```python
from build123d import *

# Parameters (mm, degrees)
F0_W         = 95.0192604214
F0_H         = 18.9093053341
F1_DEPTH     = 1.6002
F2_R         = 1.27
F3_DEPTH     = 25.4
F4_R         = 1.27
F5_DEPTH     = 2.54
F6_W         = 48.927821219
F6_H         = 30.7276230305
F7_DEPTH     = 3.6195
F8_T1_DEPTH  = 30.6197
F8_T6_DEPTH  = 56.1276230305
F8_T12_DEPTH = 56.1276230305
F8_T18_DEPTH = 56.1276230305
F8_T25_DEPTH = 56.1276230305
F8_T31_DEPTH = 56.1276230305
F8_T37_DEPTH = 56.1276230305
F8_T43_DEPTH = 56.1276230305
F8_T49_DEPTH = 56.1276230305
F8_T56_DEPTH = 56.1276230305
F8_T62_DEPTH = 56.1276230305
F9_T1_DEPTH  = 37.4142992276
F10_R        = 12.7


# Not quite as in the source:
# - a fillet or chamfer that OpenCascade refuses, or shapes differently, is made with other operations: its cross-section is extruded or revolved along the edge and cut away or added


with BuildPart() as f1:
    # F0 (on Top) → F1 (new body)
    with BuildSketch(Plane.XY):
        Polygon((-24.4639106095, -15.3638115153), (24.4639106095, -15.3638115153), (24.4639106095, -9.454652667), (24.4639106095, 9.454652667), (24.4639106095, 15.3638115153), (-24.4639106095, 15.3638115153), (-24.4639106095, 9.454652667), (-24.4639106095, -9.454652667), align=None)
        with Locations((71.9735408202, 0)):
            Rectangle(F0_W, F0_H)
        with Locations((-71.9735408202, 0)):
            Rectangle(F0_W, F0_H)
    extrude(amount=F1_DEPTH)

    # F2 (on face) → F3 (cut)
    with BuildSketch(Plane.XY.offset(1.6002)):
        with Locations((106.7831710309, 0)):
            Circle(F2_R)
        with Locations((94.0831710309, 0)):
            Circle(F2_R)
        with Locations((81.3831710309, 0)):
            Circle(F2_R)
        with Locations((68.6831710309, 0)):
            Circle(F2_R)
        with Locations((55.9831710309, 0)):
            Circle(F2_R)
        with Locations((43.2831710309, 0)):
            Circle(F2_R)
    extrude(amount=-F3_DEPTH, mode=Mode.SUBTRACT)

    # F4 (on face) → F5 (join)
    with BuildSketch(Plane.XY.offset(1.6002)):
        with Locations((-106.7719441229, 0)):
            Circle(F4_R)
        with Locations((-94.0719441229, 0)):
            Circle(F4_R)
        with Locations((-81.3719441229, 0)):
            Circle(F4_R)
        with Locations((-68.6719441229, 0)):
            Circle(F4_R)
        with Locations((-55.9719441229, 0)):
            Circle(F4_R)
        with Locations((-43.2719441229, 0)):
            Circle(F4_R)
    extrude(amount=F5_DEPTH)

    # F6 (on face) → F7 (join)
    with BuildSketch(Plane.XY.offset(1.6002)):
        Rectangle(F6_W, F6_H)
    extrude(amount=F7_DEPTH)

    # F8: fillet of radius 5.08 on 6 edges, made by hand

    # F8_s2 → F8_t1 (cut)
    with BuildSketch(Plane.XY.offset(-12.7)):
        with BuildLine():
            ThreePointArc((-19.3839106095, 15.3638115153), (-22.9760130579, 13.8759139637), (-24.4639106095, 10.2838115153))
            Line((-24.4639106095, 10.2838115153), (-24.4639106095, 15.3638115153))
            Line((-24.4639106095, 15.3638115153), (-19.3839106095, 15.3638115153))
        make_face()
        with BuildLine():
            ThreePointArc((-19.3839106095, -15.3638115153), (-22.9760130579, -13.8759139637), (-24.4639106095, -10.2838115153))
            Line((-24.4639106095, -10.2838115153), (-24.4639106095, -15.3638115153))
            Line((-24.4639106095, -15.3638115153), (-19.3839106095, -15.3638115153))
        make_face()
        with BuildLine():
            ThreePointArc((19.3839106095, -15.3638115153), (22.9760130579, -13.8759139637), (24.4639106095, -10.2838115153))
            Line((24.4639106095, -10.2838115153), (24.4639106095, -15.3638115153))
            Line((24.4639106095, -15.3638115153), (19.3839106095, -15.3638115153))
        make_face()
        with BuildLine():
            ThreePointArc((19.3839106095, 15.3638115153), (22.9760130579, 13.8759139637), (24.4639106095, 10.2838115153))
            Line((24.4639106095, 10.2838115153), (24.4639106095, 15.3638115153))
            Line((24.4639106095, 15.3638115153), (19.3839106095, 15.3638115153))
        make_face()
    extrude(amount=F8_T1_DEPTH, mode=Mode.SUBTRACT)


with BuildPart() as f8_tool4:
    # F8_s5 → F8_t6 (new body)
    with BuildSketch(Plane.XZ.offset(28.0638115153)):
        with BuildLine():
            ThreePointArc((24.4639106095, 0.1397), (22.9760130579, 3.7318024484), (19.3839106095, 5.2197))
            Line((19.3839106095, 5.2197), (24.4639106095, 5.2197))
            Line((24.4639106095, 5.2197), (24.4639106095, 0.1397))
        make_face()
    extrude(amount=-F8_T6_DEPTH)

    split(bisect_by=Plane.XY.offset(1.6002), keep=Keep.BOTTOM)

    split(bisect_by=Plane.XZ.offset(9.454652667), keep=Keep.TOP)


with BuildPart() as f1_1:
    add(f1.part)

    # F8_t3: cut F8_tool4
    add(f8_tool4.part, mode=Mode.SUBTRACT)


with BuildPart() as f8_tool10:
    # F8_s11 → F8_t12 (new body)
    with BuildSketch(Plane.XZ.offset(28.0638115153)):
        with BuildLine():
            ThreePointArc((24.4639106095, 0.1397), (22.9760130579, 3.7318024484), (19.3839106095, 5.2197))
            Line((19.3839106095, 5.2197), (24.4639106095, 5.2197))
            Line((24.4639106095, 5.2197), (24.4639106095, 0.1397))
        make_face()
    extrude(amount=-F8_T12_DEPTH)

    split(bisect_by=Plane.XY.offset(1.6002), keep=Keep.TOP)

    split(bisect_by=Plane.XZ.offset(9.454652667), keep=Keep.TOP)


with BuildPart() as f1_2:
    add(f1_1.part)

    # F8_t9: cut F8_tool10
    add(f8_tool10.part, mode=Mode.SUBTRACT)


with BuildPart() as f8_tool16:
    # F8_s17 → F8_t18 (new body)
    with BuildSketch(Plane.XZ.offset(28.0638115153)):
        with BuildLine():
            ThreePointArc((24.4639106095, 0.1397), (22.9760130579, 3.7318024484), (19.3839106095, 5.2197))
            Line((19.3839106095, 5.2197), (24.4639106095, 5.2197))
            Line((24.4639106095, 5.2197), (24.4639106095, 0.1397))
        make_face()
    extrude(amount=-F8_T18_DEPTH)

    split(bisect_by=Plane.XY.offset(1.6002), keep=Keep.TOP)

    split(bisect_by=Plane.XZ.offset(-9.454652667), keep=Keep.TOP)

    split(bisect_by=Plane.XZ.offset(9.454652667), keep=Keep.BOTTOM)


with BuildPart() as f1_3:
    add(f1_2.part)

    # F8_t15: cut F8_tool16
    add(f8_tool16.part, mode=Mode.SUBTRACT)


with BuildPart() as f8_tool23:
    # F8_s24 → F8_t25 (new body)
    with BuildSketch(Plane.XZ.offset(28.0638115153)):
        with BuildLine():
            ThreePointArc((24.4639106095, 0.1397), (22.9760130579, 3.7318024484), (19.3839106095, 5.2197))
            Line((19.3839106095, 5.2197), (24.4639106095, 5.2197))
            Line((24.4639106095, 5.2197), (24.4639106095, 0.1397))
        make_face()
    extrude(amount=-F8_T25_DEPTH)

    split(bisect_by=Plane.XY.offset(1.6002), keep=Keep.BOTTOM)

    split(bisect_by=Plane.XZ.offset(-9.454652667), keep=Keep.BOTTOM)


with BuildPart() as f1_4:
    add(f1_3.part)

    # F8_t22: cut F8_tool23
    add(f8_tool23.part, mode=Mode.SUBTRACT)


with BuildPart() as f8_tool29:
    # F8_s30 → F8_t31 (new body)
    with BuildSketch(Plane.XZ.offset(28.0638115153)):
        with BuildLine():
            ThreePointArc((24.4639106095, 0.1397), (22.9760130579, 3.7318024484), (19.3839106095, 5.2197))
            Line((19.3839106095, 5.2197), (24.4639106095, 5.2197))
            Line((24.4639106095, 5.2197), (24.4639106095, 0.1397))
        make_face()
    extrude(amount=-F8_T31_DEPTH)

    split(bisect_by=Plane.XY.offset(1.6002), keep=Keep.TOP)

    split(bisect_by=Plane.XZ.offset(-9.454652667), keep=Keep.BOTTOM)


with BuildPart() as f1_5:
    add(f1_4.part)

    # F8_t28: cut F8_tool29
    add(f8_tool29.part, mode=Mode.SUBTRACT)


with BuildPart() as f8_tool35:
    # F8_s36 → F8_t37 (new body)
    with BuildSketch(Plane.XZ.offset(-28.0638115153)):
        with BuildLine():
            ThreePointArc((-19.3839106095, 5.2197), (-22.9760130579, 3.7318024484), (-24.4639106095, 0.1397))
            Line((-24.4639106095, 0.1397), (-24.4639106095, 5.2197))
            Line((-24.4639106095, 5.2197), (-19.3839106095, 5.2197))
        make_face()
    extrude(amount=F8_T37_DEPTH)

    split(bisect_by=Plane.XZ.offset(-9.454652667), keep=Keep.BOTTOM)

    split(bisect_by=Plane.XY.offset(1.6002), keep=Keep.TOP)


with BuildPart() as f1_6:
    add(f1_5.part)

    # F8_t34: cut F8_tool35
    add(f8_tool35.part, mode=Mode.SUBTRACT)


with BuildPart() as f8_tool41:
    # F8_s42 → F8_t43 (new body)
    with BuildSketch(Plane.XZ.offset(-28.0638115153)):
        with BuildLine():
            ThreePointArc((-19.3839106095, 5.2197), (-22.9760130579, 3.7318024484), (-24.4639106095, 0.1397))
            Line((-24.4639106095, 0.1397), (-24.4639106095, 5.2197))
            Line((-24.4639106095, 5.2197), (-19.3839106095, 5.2197))
        make_face()
    extrude(amount=F8_T43_DEPTH)

    split(bisect_by=Plane.XZ.offset(-9.454652667), keep=Keep.BOTTOM)

    split(bisect_by=Plane.XY.offset(1.6002), keep=Keep.BOTTOM)


with BuildPart() as f1_7:
    add(f1_6.part)

    # F8_t40: cut F8_tool41
    add(f8_tool41.part, mode=Mode.SUBTRACT)


with BuildPart() as f8_tool47:
    # F8_s48 → F8_t49 (new body)
    with BuildSketch(Plane.XZ.offset(-28.0638115153)):
        with BuildLine():
            ThreePointArc((-19.3839106095, 5.2197), (-22.9760130579, 3.7318024484), (-24.4639106095, 0.1397))
            Line((-24.4639106095, 0.1397), (-24.4639106095, 5.2197))
            Line((-24.4639106095, 5.2197), (-19.3839106095, 5.2197))
        make_face()
    extrude(amount=F8_T49_DEPTH)

    split(bisect_by=Plane.XZ.offset(-9.454652667), keep=Keep.TOP)

    split(bisect_by=Plane.XY.offset(1.6002), keep=Keep.TOP)

    split(bisect_by=Plane.XZ.offset(9.454652667), keep=Keep.BOTTOM)


with BuildPart() as f1_8:
    add(f1_7.part)

    # F8_t46: cut F8_tool47
    add(f8_tool47.part, mode=Mode.SUBTRACT)


with BuildPart() as f8_tool54:
    # F8_s55 → F8_t56 (new body)
    with BuildSketch(Plane.XZ.offset(-28.0638115153)):
        with BuildLine():
            ThreePointArc((-19.3839106095, 5.2197), (-22.9760130579, 3.7318024484), (-24.4639106095, 0.1397))
            Line((-24.4639106095, 0.1397), (-24.4639106095, 5.2197))
            Line((-24.4639106095, 5.2197), (-19.3839106095, 5.2197))
        make_face()
    extrude(amount=F8_T56_DEPTH)

    split(bisect_by=Plane.XY.offset(1.6002), keep=Keep.TOP)

    split(bisect_by=Plane.XZ.offset(9.454652667), keep=Keep.TOP)


with BuildPart() as f1_9:
    add(f1_8.part)

    # F8_t53: cut F8_tool54
    add(f8_tool54.part, mode=Mode.SUBTRACT)


with BuildPart() as f8_tool60:
    # F8_s61 → F8_t62 (new body)
    with BuildSketch(Plane.XZ.offset(-28.0638115153)):
        with BuildLine():
            ThreePointArc((-19.3839106095, 5.2197), (-22.9760130579, 3.7318024484), (-24.4639106095, 0.1397))
            Line((-24.4639106095, 0.1397), (-24.4639106095, 5.2197))
            Line((-24.4639106095, 5.2197), (-19.3839106095, 5.2197))
        make_face()
    extrude(amount=F8_T62_DEPTH)

    split(bisect_by=Plane.XY.offset(1.6002), keep=Keep.BOTTOM)

    split(bisect_by=Plane.XZ.offset(9.454652667), keep=Keep.TOP)


with BuildPart() as f1_10:
    add(f1_9.part)

    # F8_t59: cut F8_tool60
    add(f8_tool60.part, mode=Mode.SUBTRACT)

    # F9: fillet of radius 5.08 on 2 edges, made by hand

    # F9_s2 → F9_t1 (cut)
    with BuildSketch(Plane.XZ.offset(-18.7071496138)):
        with BuildLine():
            ThreePointArc((115.7821722522, 1.6002), (117.7982347512, 1.1830201767), (119.4831710309, 0))
            Line((119.4831710309, 0), (119.4831710309, 1.6002))
            Line((119.4831710309, 1.6002), (115.7821722522, 1.6002))
        make_face()
        with BuildLine():
            ThreePointArc((-119.4831710309, 0), (-117.7982347512, 1.1830201767), (-115.7821722522, 1.6002))
            Line((-115.7821722522, 1.6002), (-119.4831710309, 1.6002))
            Line((-119.4831710309, 1.6002), (-119.4831710309, 0))
        make_face()
    extrude(amount=F9_T1_DEPTH, mode=Mode.SUBTRACT)

    # F10
    f10_edges = [f1_10.edges().sort_by_distance(p)[0] for p in [
        (24.249436, 0, 1.6002),
        (-24.249436, 0, 1.6002),
    ]]
    fillet(f10_edges, radius=F10_R)


solid = f1_10.part
```
The listing builds one solid part. Answer for the finished solid, in the listing's coordinates (mm). A direction names the side the tool comes from. Round coordinates to 2 decimals unless told otherwise and drop trailing zeros. Loops run counter-clockwise (first coordinate to the right, second up) from the corner with the lowest first, then second, coordinate; pieces in that order, holes last.
Q1. Find the intervals of material crossed by line 1 (Z direction, x = 33.5, y = -2.5); line 2 (X direction, y = -5, z = 4.2); line 3 (Y direction, x = 88.5, z = 0.65), in increasing order.
Q2. Section A-A, the plane y = 7.5 is taken. Determine the outline of the cut face in (x, z).
Q3. Which of the six approach directions +Z, -Z, +X, -X, +Y, -Y give full straight-line access (tool end or side, diameter ignored) to faces 1 (the face through (72, 0, 1.6)), 2 (the face through (-21.48, 0.215, 4.767)), 3 (the face through (22.25, 14.48, 1.99))?
Q4. Given pin 1 Ø9.5 at (x, y) = (-61.5, -3.5) entering from +Z; pin 2 Ø1.3 at (x, y) = (-94, 0) entering from +Z; pin 3 Ø6 at (x, y) = (-15, 7.5) entering from -Z; pin 4 Ø2 at (y, z) = (-5, 4.5) entering from +X, each flat-ended and moving along its own axis, determine where each tip first touches the part or whether it passes through.
Q5. Section C-C, the plane x = 47 is taken. Determine the outline of the cut face in (y, z).
Q6. Section B-B, the plane z = 2.9 is taken. Determine the outline of the cut face in (x, y).
Q7. Section D-D, the plane x = -26.5 is taken. Determine the outline of the cut face in (y, z).
Completed:
1. line 1: z = 0 to 1.6
1. line 2: x = -22.44 to 22.44
1. line 3: y = -9.45 to 9.45
2. outline: (-119.48, 0) - (119.48, 0) arc R5.08 ccw to (115.78, 1.6) - (30.14, 1.6) arc R12.7 cw to (22.46, 4.19) arc R5.08 ccw to (19.38, 5.22) - (-19.38, 5.22) arc R5.08 ccw to (-22.46, 4.19) arc R12.7 cw to (-30.14, 1.6) - (-115.78, 1.6) arc R5.08 ccw to start
3. face 1: +Z, +X, +Y, -Y
3. face 2: +Z, -X
3. face 3: +Z, -Z, +X, +Y
4. pin 1: stops at z = 1.6
4. pin 2: stops at z = 4.14
4. pin 3: stops at z = 0
4. pin 4: stops at x = 23.45
5. outline: (-9.45, 0) - (9.45, 0) - (9.45, 1.6) - (-9.45, 1.6) - close
6. outline: circle Ø2.54 at (-106.77, 0); circle Ø2.54 at (-94.07, 0); circle Ø2.54 at (-81.37, 0); circle Ø2.54 at (-68.67, 0); circle Ø2.54 at (-55.97, 0); circle Ø2.54 at (-43.27, 0); (-24.54, -9.45) - (-23.65, -9.45) - (-23.65, -13.04) arc R5.08 ccw to (-19.38, -15.36) - (19.38, -15.36) arc R5.08 ccw to (23.65, -13.04) - (23.65, -9.45) - (24.54, -9.45) - (24.54, 9.45) - (23.65, 9.45) - (23.65, 13.04) arc R5.08 ccw to (19.38, 15.36) - (-19.38, 15.36) arc R5.08 ccw to (-23.65, 13.04) - (-23.65, 9.45) - (-24.54, 9.45) - close
7. outline: (-9.45, 0) - (9.45, 0) - (9.45, 2.13) - (-9.45, 2.13) - close
